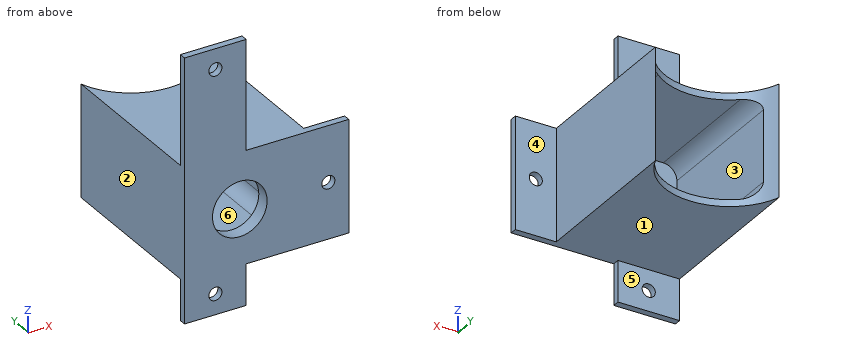
Autodesk Inventor part; units mm, degrees
ref_plane "YZ Plane" through (0, 0, 0) normal (1, 0, 0) x (0, 1, 0)
ref_plane "XZ Plane" through (0, 0, 0) normal (0, 1, 0) x (-1, 0, 0)
ref_plane "XY Plane" through (0, 0, 0) normal (0, 0, 1) x (1, 0, 0)
sketch "Sketch1" plane through (0, 0, 0) normal (0, 1, 0) x (-1, 0, 0)
  line L0 (-14.3278, -13.0048) -> (14.3278, -13.0048)
  line L1 (14.3278, -13.0048) -> (14.3278, 13.0048)
  line L2 (14.3278, 13.0048) -> (-14.3278, 13.0048)
  line L3 (-14.3278, 13.0048) -> (-14.3278, -13.0048)
  line L4 (-14.3278, -13.0048) -> (14.3278, 13.0048) construction
  line L5 (14.3278, -13.0048) -> (-14.3278, 13.0048) construction
  point P0 (0, 0)
  dimension "d0" = 28.6557
  dimension "d1" = 26.0096
extrude "Extrusion1" add sketch "Sketch1" along normal blind 40.1371
shell "Shell1" thickness 1.5875 removed faces 2 at (4.7759, 0, 4.3349) at (4.7759, 40.1371, 4.3349)
sketch "Sketch2" plane through (0, 0, 0) normal (0, 0, 1) x (1, 0, 0)
  line L0 (0, 0) -> (0, 44.45)
  circle A0 centre (0, 44.45) radius 15.113
  dimension "d5" = 44.45
  dimension "d6" = 30.226
extrude "Extrusion2" cut sketch "Sketch2" along normal mid plane 39.1617
sketch "Sketch4" plane through (-14.3278, 0, -13.0048) normal (-1, 0, 0) x (0, 0, 1)
  line L0 (26.0096, 0) -> (26.0096, 39.6421)
  line L1 (0, 0) -> (26.0096, 0)
  line L2 (26.0096, 0) -> (26.0096, 3.175)
  line L3 (26.0096, 3.175) -> (0, 3.175)
  line L4 (0, 3.175) -> (0, 0)
  point P0 (13.0048, 0)
extrude "Extrusion4" [suppressed]
sketch "Sketch5" plane through (0, 0, 0) normal (0, -1, 0) x (1, 0, 0)
  line L0 (12.7403, 11.4173) -> (-12.7403, 11.4173)
  line L1 (-12.7403, 11.4173) -> (-12.7403, -11.4173)
  line L2 (-12.7403, -11.4173) -> (12.7403, -11.4173)
  line L3 (12.7403, -11.4173) -> (12.7403, 11.4173)
  point P0 (0, 0)
extrude "Extrusion5" add sketch "Sketch5" against normal blind 3.175
sketch "Sketch6" plane through (0, 0, 0) normal (0, -1, 0) x (1, 0, 0)
  line L0 (0, 0) -> (-1.4907, 0)
  circle A0 centre (-1.4907, 0) radius 6.35
  dimension "d22" = 1.4907
  dimension "d23" = 12.7
extrude "Extrusion6" cut sketch "Sketch6" against normal blind 3.175
fillet "Fillet1" radius 3.175 4 edges at (-12.7403, 19.7478, -11.4173) (-12.7403, 19.7478, 11.4173) (12.7403, 19.7478, 11.4173) (12.7403, 19.7478, -11.4173)
sketch "Sketch11" plane through (14.3278, 0, 13.0048) normal (1, 0, 0) x (0, 0, -1)
  line L0 (0, 0) -> (0, 39.6421)
  line L1 (26.0096, 0) -> (26.0096, 39.6421)
  line L2 (0, 0) -> (26.0096, 0)
  line L3 (26.0096, 0) -> (26.0096, 1.5875)
  line L4 (26.0096, 1.5875) -> (0, 1.5875)
  line L5 (0, 1.5875) -> (0, 0)
  point P0 (13.0048, 0)
  dimension "d36" = 1.5875
extrude "Extrusion11" add sketch "Sketch11" along normal blind 9.525
sketch "Sketch12" plane through (0, 44.45, -13.0048) normal (0, 0, -1) x (-1, 0, 0)
  line L0 (-23.8528, -44.45) -> (14.3278, -44.45)
  line L1 (0, -44.45) -> (0, -42.8625)
  line L2 (14.3278, -44.45) -> (0, -44.45)
  line L3 (0, -44.45) -> (0, -42.8625)
  line L4 (0, -42.8625) -> (14.3278, -42.8625)
  line L5 (14.3278, -42.8625) -> (14.3278, -44.45)
  dimension "d39" = 1.5875
extrude "Extrusion12" add sketch "Sketch12" along normal blind 9.525
sketch "Sketch13" plane through (0, 44.45, 13.0048) normal (0, 0, 1) x (1, 0, 0)
  point P0 (0, -44.45)
sketch "Sketch14" plane through (-14.3278, 0, 13.0048) normal (-1, 0, 0) x (0, 0, 1)
  point P0 (-13.0048, 0)
sketch "Sketch15" plane through (0, 44.45, 13.0048) normal (0, 0, 1) x (1, 0, 0)
  line L0 (-14.3278, -44.45) -> (23.8528, -44.45)
  line L1 (-14.3278, -44.45) -> (0, -44.45)
  line L2 (0, -44.45) -> (0, -42.8625)
  line L3 (0, -42.8625) -> (-14.3278, -42.8625)
  line L4 (-14.3278, -42.8625) -> (-14.3278, -44.45)
  point P0 (0, -44.45)
  dimension "d42" = 1.5875
extrude "Extrusion13" add sketch "Sketch15" along normal blind 25.4
sketch "Sketch16" plane through (-14.3278, 1.5875, -13.0048) normal (0, 1, 0) x (1, 0, 0)
  line L0 (14.3278, 0) -> (14.3278, 9.525)
  line L1 (0, -51.4096) -> (0, 9.525)
  line L2 (14.3278, 9.525) -> (0, 9.525)
  line L3 (14.3278, -26.0096) -> (14.3278, -51.4096)
  line L4 (38.1807, -26.0096) -> (38.1807, 0)
  line L5 (14.3278, -26.0096) -> (38.1807, -26.0096)
  line L6 (38.1807, 0) -> (14.3278, 0)
  line L7 (38.1807, 0) -> (33.4182, 0)
  circle A0 centre (7.1639, 4.7625) radius 1.524
  circle A1 centre (33.4182, -13.0048) radius 1.524
  circle A2 centre (7.1639, -46.6471) radius 1.524
  point P0 (14.3278, -13.0048)
  dimension "d45" = 4.7625
  dimension "d47" = 3.048
  dimension "d48" = 3.048
  dimension "d63" = 3.048
extrude "Extrusion14" cut sketch "Sketch16" against normal blind 25.4
properties part number "DPLX_P016_Spark_Gap_Camera_Shroud"
For this review, take the finished solid that the model builds, in its own axes (mm). Face numbers are marked on the shaded views. A direction names the side the tool comes from. Round coordinates to 2 decimals unless told otherwise and drop trailing zeros. Write each loop counter-clockwise with the first axis right and the second up, starting at its lowest first coordinate (ties: lowest second). Pieces come first, ordered by that corner, then holes. Notation, with made-up numbers: M 77,31.25 L 114,31.25 A14 ccw 114,35.25 Z; hole C -32,-20.5 d6. An arc over 180 degrees is marked long. One line per item, written item: value. Start each with the question number.
(1) We need section B-B (z = 0). Count the separate pieces of the cut face and the enclosed holes in it, and give its area (3 significant figures).
(2) Insertion check: pin 1 (7.5 mm diameter, centred on x = -1.49, z = 0, fed in from +Y); pin 2 (4.5 mm diameter, centred on x = -8.5, z = 21, fed in from +Y); pin 3 (6 mm diameter, centred on x = 3.5, y = 18.5, fed in from -Z); pin 4 (11.5 mm diameter, centred on x = 3.5, z = 2.5, fed in from +Y) (3 decimals). Each pin has a flat end and moves straight along its axis. Give the tip position at first contact, or say it passes through.
(3) The part is to be moulded in two halves that separate along X. For the marked faces 1, 2 and 3, say which applies: released by +X, released by -X, zero draft, split by the parting line, or undercut.
(4) We need section D-D (z = 29). Give the boundary of the cut face in (x, y), and give its area (3 significant figures).
(5) Wall thickness on line 1 (Z direction, x = -3, y = 15.5); line 2 (X direction, y = 26, z = -6); line 3 (Y direction, x = -12, z = 24): over which ranges is each line inside the solid? List them lowest first.
(6) We need section C-C (x = 8.5). Give the boundary of the cut face in (y, z) (3 decimals), and give its area (3 significant figures).
(7) We need section A-A (y = 27). Give the boundary of the cut face in (x, z) (3 decimals).
(8) Machinability: for the marked faces 4, 5 and 6, which of the approach directions +Z, -Z, +X, -X, +Y, -Y give a long, thin tool a straight path to every point of the face, cutting with its end or side? Answer none if there is none.
Result:
1. separate pieces: 3
1. enclosed holes: 0
1. area: 171 mm²
2. pin 1: through
2. pin 2: y = 1.59
2. pin 3: z = -13
2. pin 4: y = 3.175
3. face 1: zero draft
3. face 2: released by -X
3. face 3: undercut
4. outline: M -14.33,0 L 0,0 L 0,1.59 L -14.33,1.59 Z
4. area: 22.7 mm²
5. line 1: -13 to -11.42, 11.42 to 13
5. line 2: -14.33 to -12.74, 12.74 to 14.33
5. line 3: 0 to 1.59
6. outline: M 0,-13.005 L 31.954,-13.005 L 31.954,-11.417 L 3.175,-11.417 L 3.175,11.417 L 31.954,11.417 L 31.954,13.005 L 0,13.005 Z
6. area: 174 mm²
7. outline: M -14.328,-13.005 L 14.328,-13.005 L 14.328,13.005 L -14.328,13.005 Z; hole M -12.74,-8.242 A3.175 ccw -9.565,-11.417 L 9.565,-11.417 A3.175 ccw 12.74,-8.242 L 12.74,8.242 A3.175 ccw 9.565,11.417 L -9.565,11.417 A3.175 ccw -12.74,8.242 Z
8. face 4: +Z, -Z, +X, +Y
8. face 5: -Z, +X, -X, +Y
8. face 6: +Y
